Verification items for the finished model (mm, model axes). Face numbers are marked on the shaded views. A direction names the side the tool comes from. Give positions to 0.01 mm unless a question says otherwise; leave off trailing zeros. Loops run counter-clockwise (first coordinate to the right, second up) from the corner with the lowest first, then second, coordinate; pieces in that order, holes last. Notation, with made-up numbers: M 5.25,-9 L 17.25,-9 A24 ccw 17.25,28 Z; hole C 13,-30 d11. An arc over 180 degrees is marked long. Use CSV: the item, a comma, the result in double quotes.
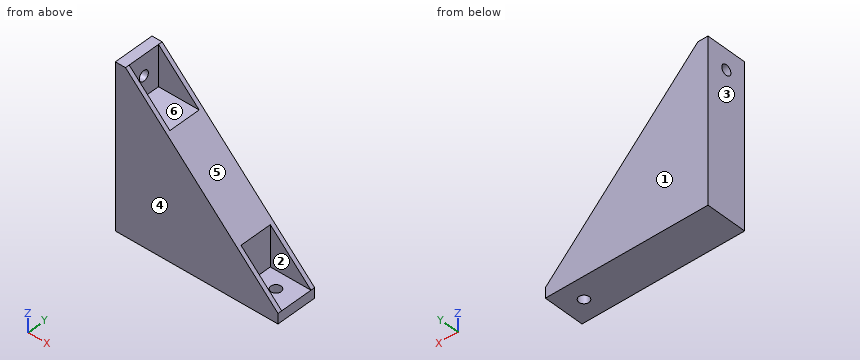
Autodesk Inventor part; units mm, degrees
ref_plane "YZ Plane" through (0, 0, 0) normal (1, 0, 0) x (0, 1, 0)
ref_plane "XZ Plane" through (0, 0, 0) normal (0, 1, 0) x (-1, 0, 0)
ref_plane "XY Plane" through (0, 0, 0) normal (0, 0, 1) x (1, 0, 0)
sketch "Sketch1" plane through (0, 0, 0) normal (0, 0, 1) x (1, 0, 0)
  line L0 (0, 0) -> (80, 0)
  line L1 (80, 0) -> (80, 20)
  line L2 (80, 20) -> (0, 20)
  line L3 (0, 20) -> (0, 0)
  circle A0 centre (70, 10) radius 2.5
  point P0 (80, 10)
  dimension "d0" = 80
  dimension "d1" = 20
  dimension "d2" = 5
  dimension "d3" = 10
extrude "Extrusion1" add sketch "Sketch1" along normal blind 5
sketch "Sketch2" plane through (0, 0, 0) normal (-1, 0, 0) x (0, 0, 1)
  line L0 (0, 0) -> (0, 20)
  line L1 (0, 20) -> (80, 20)
  line L2 (80, 20) -> (80, 0)
  line L3 (80, 0) -> (0, 0)
  line L4 (0, 0) -> (0, 20)
  circle A0 centre (70, 10) radius 2.5
  point P0 (5, 0)
  point P1 (80, 10)
  dimension "d6" = 80
  dimension "d7" = 5
  dimension "d8" = 10
extrude "Extrusion2" add sketch "Sketch2" against normal blind 5
sketch "Sketch3" plane through (0, 20, 0) normal (0, 1, 0) x (1, 0, 0)
  line L0 (80, -5) -> (5, -5)
  line L1 (5, -5) -> (5, -80)
  line L2 (5, -80) -> (5, -5)
  line L3 (5, -80) -> (80, -5)
  point P0 (0, 0)
extrude "Extrusion3" add sketch "Sketch3" against normal blind 2
sketch "Sketch4" plane through (0, 0, 0) normal (0, -1, 0) x (1, 0, 0)
  line L0 (80, 5) -> (5, 5)
  line L1 (80, 5) -> (5, 80)
  line L2 (5, 5) -> (5, 80)
  point P0 (0, 0)
extrude "Extrusion4" add sketch "Sketch4" against normal blind 2
sketch "Sketch5" plane through (0, 18, 0) normal (0, -1, 0) x (1, 0, 0)
  line L0 (5, 72.5) -> (5, 67.5)
  line L1 (67.5, 5) -> (72.5, 5)
  line L2 (5, 67.5) -> (5, 5)
  line L3 (5, 5) -> (67.5, 5)
  line L4 (5, 60) -> (60, 5)
  line L5 (70, 5) -> (70, 0)
  line L6 (80, 0) -> (0, 0)
  line L7 (5, 70) -> (0, 70)
  line L8 (5, 60) -> (25, 60)
  line L9 (60, 5) -> (60, 25)
  line L10 (5, 80) -> (80, 5)
  line L11 (25, 60) -> (60, 25)
  dimension "d15" = 10
  dimension "d16" = 10
extrude "Extrusion5" add sketch "Sketch5" along normal blind 16
properties part number "L Bracket Small"
(1) Section check D-D on y = 15.75. Record the cut outline in (x, z), plus the area to 3 significant figures.
Calculated:
outline,"M 0,0 L 80,0 L 80,5 L 60,5 L 60,25 L 25,60 L 5,60 L 5,80 L 0,80 Z"
area,"3,190 mm²"
(2) Section check B-B on z = 70. Record the cut outline in (x, y).
Calculated:
outline,"M 0,0 L 15,0 L 15,2 L 5,2 L 5,7.5 L 0,7.5 Z; M 0,12.5 L 5,12.5 L 5,18 L 15,18 L 15,20 L 0,20 Z"
(3) Section check C-C on y = 10. Record the cut outline in (x, z).
Calculated:
outline,"M 0,0 L 67.5,0 L 67.5,5 L 60,5 L 60,25 L 25,60 L 5,60 L 5,67.5 L 0,67.5 Z; M 0,72.5 L 5,72.5 L 5,80 L 0,80 Z; M 72.5,0 L 80,0 L 80,5 L 72.5,5 Z"
(4) Section check A-A on x = 70. Record the cut outline in (y, z).
Calculated:
outline,"M 0,0 L 7.5,0 L 7.5,5 L 2,5 L 2,15 L 0,15 Z; M 12.5,0 L 20,0 L 20,15 L 18,15 L 18,5 L 12.5,5 Z"
(5) Tool access check on the marked faces 5 and 6. Record the directions out of +Z, -Z, +X, -X, +Y, -Y that give a thin tool (end or side, any length) a straight path to the whole face; none if there is none.
Calculated:
face 5,"+Z, +X, +Y, -Y"
face 6,"+Z, +X"
(6) Mould release check, pull along Y, two halves, no side actions. Record for the marked faces 1, 2, 3 and 4: released by +Y, released by -Y, zero draft, split by the parting line, or undercut.
Calculated:
face 1,"released by +Y"
face 2,"undercut"
face 3,"zero draft"
face 4,"released by -Y"
(7) Scan lines: L1, parallel to Y at x = 70, z = 1.15; L2, parallel to Z at x = 22.5, y = 7.5. Record each from-to range of solid material in increasing order. Write a range as from..to.
Calculated:
L1,"y = 0..7.5, 12.5..20"
L2,"z = 0..60"
(8) Depth check by flat-ended pin: pin 1 Ø5 at (y, z) = (10, 19.5) entering from +X; pin 2 Ø4.5 at (x, y) = (70, 10) entering from -Z; pin 3 Ø8 at (x, y) = (16.5, 11) entering from +Z. Enter the tip coordinate at first touch or a pass-through.
Calculated:
pin 1,"stops at x = 60"
pin 2,"passes through"
pin 3,"stops at z = 60"
